Input: dimensioned drawing with shaded views. Units: mm. Origin: part minimum x, y, z. A direction names the side the tool comes from. Round coordinates to 2 decimals unless told otherwise and drop trailing zeros. Order: outer loops, then holes, each group sorted by start corner. A loop starts at its lowest first (then second) coordinate and runs counter-clockwise, first axis right, second up. Notation, with made-up numbers: M -0.5,35 L 5.5,35 A32 cw 5.5,61 Z; hole C 28.5,75 d2. An arc over 180 degrees is marked long. One line per question, with ' | ' between items.
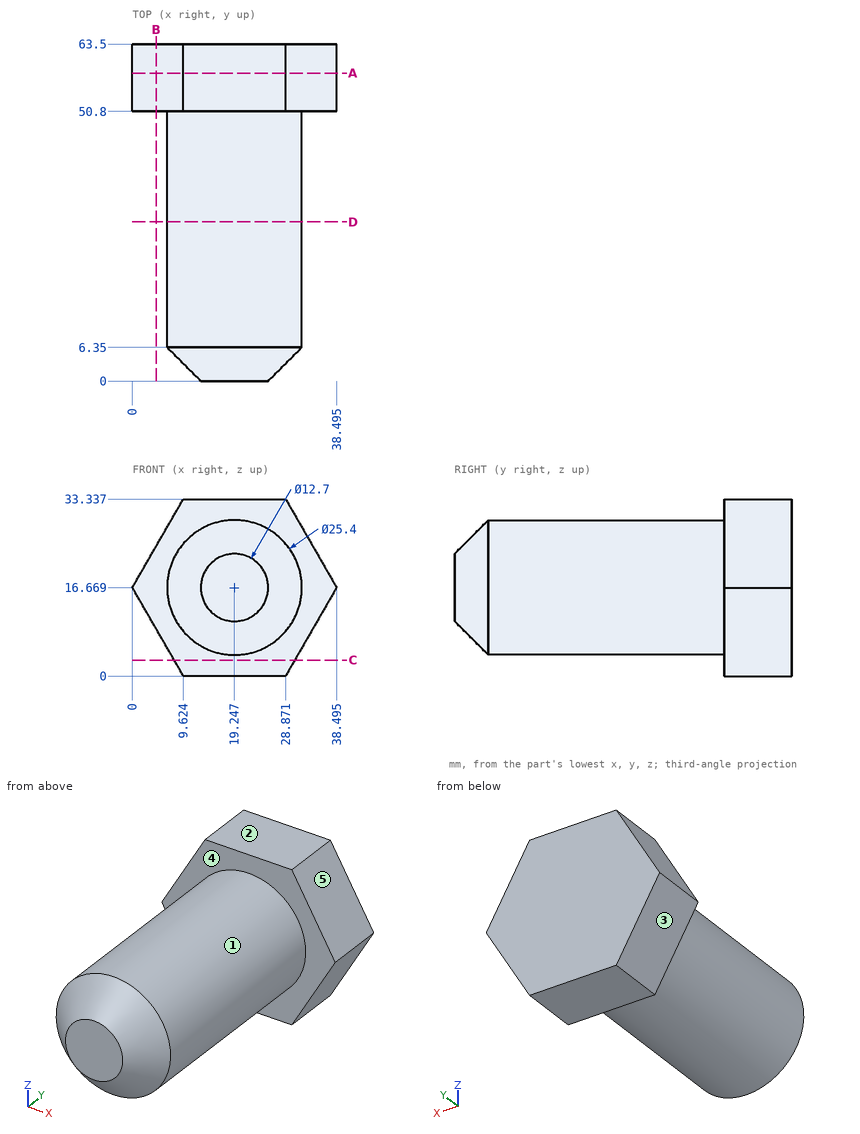
Item 1: Section query D-D, the plane y = 30. Return loops of the section in (x, z), plus the area to 3 significant figures.
Report:
outline: C 19.25,16.67 d25.4 | area: 507 mm²
Item 2: Section query C-C, the plane z = 3. Return loops of the section in (x, y).
Report:
outline: M 7.89,50.8 L 30.6,50.8 L 30.6,63.5 L 7.89,63.5 Z
Item 3: Section query A-A, the plane y = 58. Return loops of the section in (x, z) (1 decimal).
Report:
outline: M 0,16.7 L 9.6,0 L 28.9,0 L 38.5,16.7 L 28.9,33.3 L 9.6,33.3 Z
Item 4: Section query B-B, the plane x = 4.5. Return loops of the section in (y, z) (1 decimal).
Report:
outline: M 50.8,8.9 L 63.5,8.9 L 63.5,24.5 L 50.8,24.5 Z
Item 5: First-contact query: pin 1 (2 mm diameter, centred on y = 16, z = 19, fed in from +X); pin 2 (10 mm diameter, centred on x = 6, z = 26, fed in from -Y) (1 decimal); pin 3 (1.5 mm diameter, centred on y = 20.5, z = 25.5, fed in from +X) (1 decimal); pin 4 (8 mm diameter, centred on x = 9, z = 17.5, fed in from -Y). Flat tips, straight axial feed; report the tip coordinate or a pass-through.
Report:
pin 1: x = 31.88 | pin 2: y = 4.9 | pin 3: x = 29 | pin 4: y = 0
Item 6: Access query for the marked faces 4 and 5. Directions: +Z, -Z, +X, -X, +Y, -Y. A direction counts if a zero-diameter tool reaches every point of the face in a straight line with its end or side. Return the directions, or none.
Report:
face 4: -Y | face 5: +Z, +X, +Y, -Y
Item 7: Mould query, pull axis X, two halves, no side actions, for the marked faces 1, 2 and 3. Classes: +X half, -X half, draft (parallel to the pull), parting line (faces both ways), or undercut.
Report:
face 1: parting line | face 2: draft | face 3: -X half
Item 8: Line query: line 1 along Y through (x, z) = (33, 19.5); line 2 along Y through (x, z) = (26.5, 26); line 3 along X through (y, z) = (48, 19). Output: solid intervals per line, ascending. Write a range as from..to.
Report:
line 1: 50.8..63.5 | line 2: 5.47..63.5 | line 3: 6.76..31.73
